Read the model definition and answer for the solid it produces. Units are mm, in the model's axes. Face numbers are marked on the shaded views. A direction names the side the tool comes from. Round coordinates to 2 decimals unless told otherwise and drop trailing zeros. Loops run counter-clockwise (first coordinate to the right, second up) from the corner with the lowest first, then second, coordinate; pieces in that order, holes last. Notation, with made-up numbers: (-19, 26) - (-4, 26) arc R16 cw to (-4, 47) - close; hole circle Ø7 at (48, 29). An arc over 180 degrees is marked (long way). Use one line per item in the form item = value. Start each with the question number.
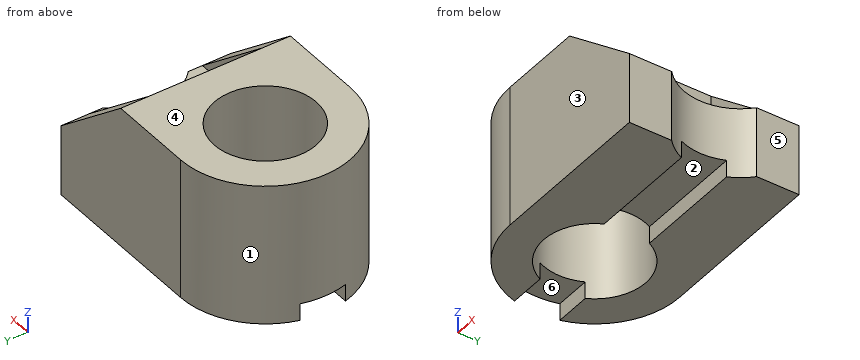
```python
from build123d import *

# Parameters (mm, degrees)
SKETCH1_R           = 18
BOSS_EXTRUDE1_DEPTH = 50
BOSS_EXTRUDE3_DEPTH = 25
BOSS_EXTRUDE4_DEPTH = 10
BOSS_EXTRUDE5_DEPTH = 10
CUT_EXTRUDE2_DEPTH  = 6
CUT_EXTRUDE3_DEPTH  = 6


with BuildPart() as part:
    # Sketch1 → Boss-Extrude1 (new body)
    with BuildSketch(Plane.XY):
        with BuildLine():
            Line((0, 30), (30, 30))
            Line((30, 30), (30, -30))
            Line((30, -30), (0, -30))
            ThreePointArc((0, -30), (-30, 0), (0, 30))
        make_face()
        Circle(SKETCH1_R, mode=Mode.SUBTRACT)
    extrude(amount=-BOSS_EXTRUDE1_DEPTH)

    # Sketch2 → Boss-Extrude3 (add)
    with BuildSketch(Plane(origin=(0, 0, -50), x_dir=(-1, 0, 0), z_dir=(0, 0, -1))):
        with BuildLine():
            Line((-60, 30), (-60, 15))
            ThreePointArc((-60, 15), (-53.228756555, 0), (-60, -15))
            Line((-60, -15), (-60, -30))
            Line((-60, -30), (-30, -30))
            Line((-30, -30), (-30, 30))
            Line((-30, 30), (-60, 30))
        make_face()
    extrude(amount=-BOSS_EXTRUDE3_DEPTH)

    # Sketch6 → Boss-Extrude4 (add)
    with BuildSketch(Plane(origin=(0, 30, 0), x_dir=(1, 0, 0), z_dir=(0, 1, 0))):
        Polygon((60, 25), (30, 0), (30, 25), align=None)
    extrude(amount=-BOSS_EXTRUDE4_DEPTH)

    # Sketch11 → Boss-Extrude5 (add)
    with BuildSketch(Plane(origin=(0, -30, 0), x_dir=(-1, 0, 0), z_dir=(0, -1, 0))):
        Polygon((-30, 0), (-30, 25), (-60, 25), align=None)
    extrude(amount=-BOSS_EXTRUDE5_DEPTH)

    # Sketch12 → Cut-Extrude2 (cut)
    with BuildSketch(Plane(origin=(0, 0, -50), x_dir=(-1, 0, 0), z_dir=(0, 0, -1))):
        with BuildLine():
            Line((28.91366459, 8), (16.124515497, 8))
            ThreePointArc((16.124515497, 8), (-18, 0), (16.124515497, -8))
            Line((16.124515497, -8), (28.91366459, -8))
            ThreePointArc((28.91366459, -8), (30, 0), (28.91366459, 8))
        make_face()
    extrude(amount=-CUT_EXTRUDE2_DEPTH, mode=Mode.SUBTRACT)

    # Sketch12_8 → Cut-Extrude3 (cut)
    with BuildSketch(Plane(origin=(0, 0, -50), x_dir=(-1, 0, 0), z_dir=(0, 0, -1))):
        with BuildLine():
            Line((-16.124515497, 8), (-54.898453775, 8))
            ThreePointArc((-54.898453775, 8), (-53.228756555, 0), (-54.898453775, -8))
            Line((-54.898453775, -8), (-16.124515497, -8))
            ThreePointArc((-16.124515497, -8), (-18, 0), (-16.124515497, 8))
        make_face()
    extrude(amount=-CUT_EXTRUDE3_DEPTH, mode=Mode.SUBTRACT)


solid = part.part
```
1) For the marked faces 5 and 6, determine the directions among +Z, -Z, +X, -X, +Y, -Y from which every point of the face is accessible in a straight line to the end or side of a thin tool.
2) A cutting plane is placed at C-C on y = 0. Write down the section's boundary in (x, z).
3) A cutting plane is placed at B-B on z = -45.5. Write down the section's boundary in (x, y), plus the area to 3 significant figures.
4) Straight lines are drawn through the part: line 1 (Y direction, x = 0, z = -18); line 2 (X direction, y = 0, z = -35); line 3 (Y direction, x = 30.5, z = -18). For each, find the intervals that lie inside material, in ascending order. Write a range as from..to.
5) A cutting plane is placed at A-A on x = 8. Write down the section's boundary in (y, z), plus the area to 3 significant figures.
6) Determine the mould class of the marked faces 1, 2, 3 and 4 for opening direction Y: +Y half, -Y half, draft (parallel to the pull), parting line (faces both ways), or undercut.
7) A cutting plane is placed at D-D on z = -27. Write down the section's boundary in (x, y), plus the area to 3 significant figures.
8) Flat-ended cylindrical pins translate along their axes: pin 1 (4 mm diameter, centred on y = -8, z = -32.5, fed in from -X); pin 2 (6.5 mm diameter, centred on x = -20.5, z = -46.5, fed in from -Y); pin 3 (12.5 mm diameter, centred on y = 4.5, z = -17.5, fed in from +X). Find the tip coordinate at first contact, or state that the pin passes through.
Checks:
q1.face_5 = +Z, -Z, +X, +Y, -Y
q1.face_6 = -Z, +X, -X
q2.outline = (-30, -44) - (-18, -44) - (-18, 0) - (-30, 0) - close; (18, -44) - (53.23, -44) - (53.23, -25) - (30, -25) - (30, 0) - (18, 0) - close
q3.outline = (-28.91, -8) arc R30 ccw to (0, -30) - (60, -30) - (60, -15) arc R20 cw to (54.9, -8) - (16.12, -8) arc R18 cw to (-16.12, -8) - close; (-28.91, 8) - (-16.12, 8) arc R18 cw to (16.12, 8) - (54.9, 8) arc R20 cw to (60, 15) - (60, 30) - (0, 30) arc R30 ccw to start
q3.area = 3,080 mm²
q4.line_1 = -30..-18, 18..30
q4.line_2 = -30..-18, 18..53.23
q4.line_3 = -30..-20, 20..30
q5.outline = (-30, -50) - (-16.12, -50) - (-16.12, 0) - (-30, 0) - close; (16.12, -50) - (30, -50) - (30, 0) - (16.12, 0) - close
q5.area = 1,390 mm²
q6.face_1 = parting line
q6.face_2 = undercut
q6.face_3 = -Y half
q6.face_4 = draft
q7.outline = (0, -30) - (60, -30) - (60, -15) arc R20 cw to (60, 15) - (60, 30) - (0, 30) arc R30 ccw to start; hole circle Ø36 at (0, 0)
q7.area = 3,860 mm²
q8.pin_1 = -29.39
q8.pin_2 = -24.54
q8.pin_3 = 30
